```python
from build123d import *

# Parameters (mm, degrees)
ESQUISSE2_W             = 100
ESQUISSE2_H             = 210
BOSS_EXTRU_1_DEPTH      = 10
ESQUISSE3_W             = 20
ESQUISSE3_H             = 35
ENL_V_MAT_EXTRU_1_DEPTH = 10
ESQUISSE4_R             = 1.5
ENL_V_MAT_EXTRU_2_DEPTH = 10
ESQUISSE6_R             = 1.5
ENL_V_MAT_EXTRU_3_DEPTH = 10


with BuildPart() as part:
    # Esquisse2 → Boss.-Extru.1 (new body)
    with BuildSketch(Plane.XY):
        with Locations((50, 105)):
            Rectangle(ESQUISSE2_W, ESQUISSE2_H)
    extrude(amount=BOSS_EXTRU_1_DEPTH)

    # Esquisse3 → Enlèv. mat.-Extru.1 (cut)
    with BuildSketch(Plane.XY):
        with Locations((10, 192.5)):
            Rectangle(ESQUISSE3_W, ESQUISSE3_H)
        with Locations((10, 17.5)):
            Rectangle(ESQUISSE3_W, ESQUISSE3_H)
    extrude(amount=ENL_V_MAT_EXTRU_1_DEPTH, mode=Mode.SUBTRACT)

    # Esquisse4 → Enlèv. mat.-Extru.2 (cut)
    with BuildSketch(Plane(origin=(0, 0, 0), x_dir=(-1, 0, 0), z_dir=(0, 0, -1))):
        with Locations((-25, 200)):
            Circle(ESQUISSE4_R)
        with Locations((-60, 200)):
            Circle(ESQUISSE4_R)
        with Locations((-25, 10)):
            Circle(ESQUISSE4_R)
        with Locations((-60, 10)):
            Circle(ESQUISSE4_R)
    extrude(amount=-ENL_V_MAT_EXTRU_2_DEPTH, mode=Mode.SUBTRACT)

    # Esquisse6 → Enlèv. mat.-Extru.3 (cut)
    with BuildSketch(Plane(origin=(0, 0, 0), x_dir=(-1, 0, 0), z_dir=(0, 0, -1))):
        with Locations((-25.645889501, 130.633743079)):
            Circle(ESQUISSE6_R)
        with Locations((-25.645889501, 79.385925673)):
            Circle(ESQUISSE6_R)
        with Locations((-67.742251285, 79.385925673)):
            Circle(ESQUISSE6_R)
        with Locations((-66.161997433, 130.633743079)):
            Circle(ESQUISSE6_R)
    extrude(amount=-ENL_V_MAT_EXTRU_3_DEPTH, mode=Mode.SUBTRACT)


solid = part.part
```
Could you check a few things on this model? Use its own coordinates, in mm. A direction names the side the tool comes from. Round coordinates to 2 decimals unless told otherwise and drop trailing zeros. Loops run counter-clockwise (first coordinate to the right, second up) from the corner with the lowest first, then second, coordinate; pieces in that order, holes last. Notation, with made-up numbers: M 46.25,39.25 L 84.25,39.25 A14 cw 84.25,66.25 Z; hole C -37,16.5 d5. An arc over 180 degrees is marked long. Write item = value, one per line.
1. Will these pins go through, and if not, where does the flat tip stop? P1, Ø5, axis at y = 23.5, z = 7, coming from the -X side; P2, Ø2.5, axis at x = 67.74, y = 79.39, coming from the -Z side; P3, Ø5, axis at x = 11.5, z = 6.5, coming from the -Y side; P4, Ø3, axis at x = 13, z = 3, coming from the +Y side.
Results below:
P1 = 20
P2 = through
P3 = 35
P4 = 175
2. I need wall thicknesses on probe 1 along X at (y, z) = (79.5, 1); probe 2 along Y at (x, z) = (25, 7); probe 3 along Y at (x, z) = (19, 6). Which ranges of each line are inside material? Lowest first, please.
Results below:
probe_1 = 0 to 24.15, 27.14 to 66.25, 69.24 to 100
probe_2 = 0 to 8.5, 11.5 to 78.03, 80.74 to 129.28, 131.99 to 198.5, 201.5 to 210
probe_3 = 35 to 175
3. I want a section at A-A, the plane z = 5. Count the separate pieces of the cut face and the enclosed holes in it, and give its area (3 significant figures).
Results below:
separate_pieces = 1
enclosed_holes = 8
area = 19,500 mm²
4. I want a section at B-B, the plane y = 16.5. Write out the boundary of the cut face in (x, z).
Results below:
outline = M 20,0 L 100,0 L 100,10 L 20,10 Z
5. Which directions (+Z, -Z, +X, -X, +Y, -Y) give clear straight access to the entire face, cutting with the end or side of a thin tool? Please do faces 1 (the face through (20, 17, 5)), 2 (the face through (10, 175, 5)), 3 (the face through (100, 104, 5)).
Results below:
face_1 = +Z, -Z, -X, -Y
face_2 = +Z, -Z, -X, +Y
face_3 = +Z, -Z, +X, +Y, -Y
